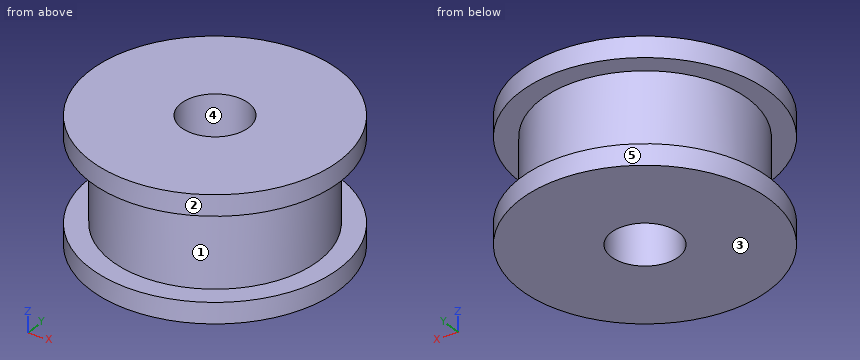
Autodesk Inventor part; units mm, degrees
ref_plane "YZ Plane" through (0, 0, 0) normal (1, 0, 0) x (0, 1, 0)
ref_plane "XZ Plane" through (0, 0, 0) normal (0, 1, 0) x (-1, 0, 0)
ref_plane "XY Plane" through (0, 0, 0) normal (0, 0, 1) x (1, 0, 0)
sketch "Sketch1" plane through (0, 0, 0) normal (0, 0, 1) x (1, 0, 0)
  circle A0 centre (0, 0) radius 10
  circle A1 centre (0, 0) radius 3.25
  dimension "d0" = 20
  dimension "d1" = 6.5
extrude "Extrusion1" add sketch "Sketch1" along normal blind 12
sketch "Sketch2" plane through (0, 0, 12) normal (0, 0, 1) x (1, 0, 0)
  circle A0 centre (0, 0) radius 12
  dimension "d4" = 24
extrude "Extrusion2" add sketch "Sketch2" against normal blind 2
sketch "Sketch3" plane through (0, 0, 12) normal (0, 0, 1) x (1, 0, 0)
  circle A0 centre (0, 0) radius 3.25
  dimension "d7" = 6.5
sketch "Sketch4" plane through (0, 0, 0) normal (0, 0, -1) x (-1, 0, 0)
  circle A0 centre (0, 0) radius 12
  circle A1 centre (0, 0) radius 10
  dimension "d8" = 24
extrude "Extrusion3" add sketch "Sketch4" against normal blind 2
extrude "Extrusion4" cut sketch "Sketch3" against normal through all
properties part number "poulie v2"
Input: part model. Units: mm. Frame: model coordinates. Face numbers are marked on the shaded views. A direction names the side the tool comes from. Coordinates: 2 decimals unless noted, no trailing zeros. Loops run counter-clockwise (first coordinate to the right, second up) from the corner with the lowest first, then second, coordinate; pieces in that order, holes last.
Q1. Section C-C, the plane z = 8.25. Return the cut outline in (x, y).
Results are:
outline: circle Ø20 at (0, 0); hole circle Ø6.5 at (0, 0)
Q2. Section A-A, the plane x = 0. Return the cut outline in (y, z).
Results are:
outline: (-12, 0) - (-3.25, 0) - (-3.25, 12) - (-12, 12) - (-12, 10) - (-10, 10) - (-10, 2) - (-12, 2) - close; (3.25, 0) - (12, 0) - (12, 2) - (10, 2) - (10, 10) - (12, 10) - (12, 12) - (3.25, 12) - close
Q3. Contact query for flat-ended pins moving along their axis: pin 1 (3 mm diameter, centred on x = 0, z = 4.5, fed in from +Y); pin 2 (1 mm diameter, centred on y = -5, z = 2, fed in from -X); pin 3 (3 mm diameter, centred on y = 4, z = 4.5, fed in from -X). Output: stop coordinate, or through.
Results are:
pin 1: stops at y = 10
pin 2: stops at x = -11.12
pin 3: stops at x = -9.68
Q4. Set-up query: the marked faces 1 and 2. Return all of +Z, -Z, +X, -X, +Y, -Y with unobstructed straight access to the full face (end or side cutting, diameter ignored); none if empty.
Results are:
face 1: none
face 2: +Z, -Z
Q5. Mould query, pull axis X, two halves, no side actions, for the marked faces 3, 4 and 5. Classes: +X half, -X half, draft (parallel to the pull), parting line (faces both ways), or undercut.
Results are:
face 3: draft
face 4: undercut
face 5: parting line
Q6. Section D-D, the plane y = -4.75. Return the cut outline in (x, z).
Results are:
outline: (-11.02, 0) - (11.02, 0) - (11.02, 2) - (8.8, 2) - (8.8, 10) - (11.02, 10) - (11.02, 12) - (-11.02, 12) - (-11.02, 10) - (-8.8, 10) - (-8.8, 2) - (-11.02, 2) - close
Q7. Line query: line 1 along Y through (x, z) = (0, 6.5); line 2 along Z through (x, y) = (-9.5, 6); line 3 along Y through (x, z) = (1, 4.5). Output: solid intervals per line, ascending.
Results are:
line 1: y = -10 to -3.25, 3.25 to 10
line 2: z = 0 to 2, 10 to 12
line 3: y = -9.95 to -3.09, 3.09 to 9.95
